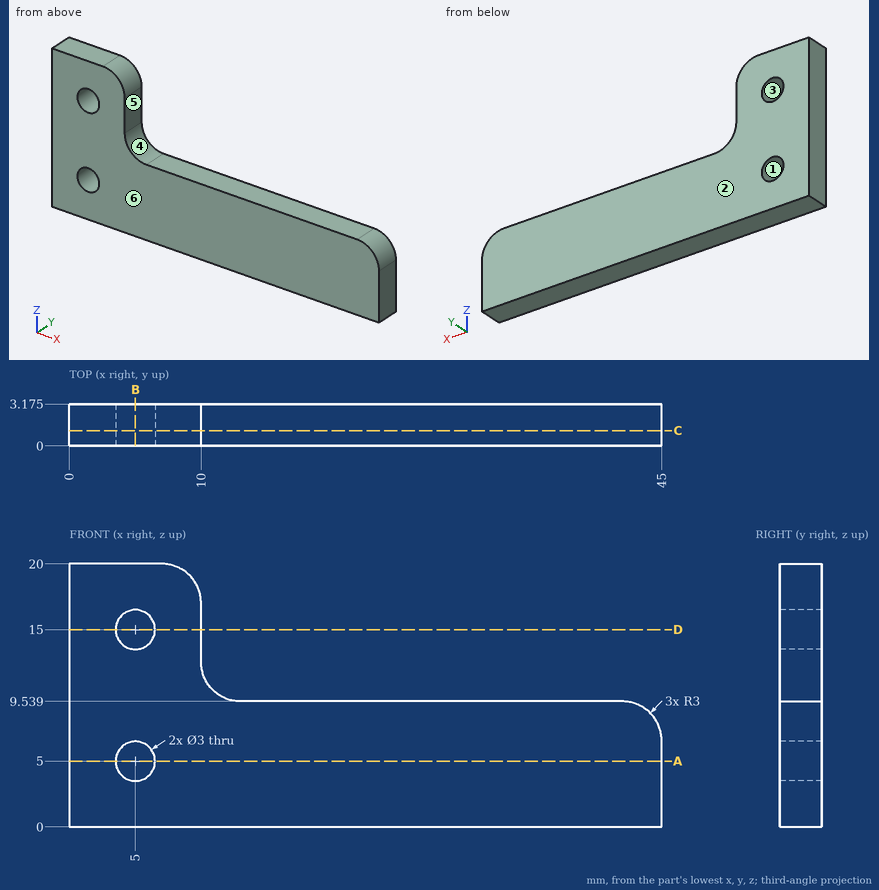
Study the drawing (mm; zero at the part's minimum x, y, z) and answer. A direction names the side the tool comes from. Give positions to 0.01 mm unless a question says otherwise; leave off trailing zeros. Write each loop counter-clockwise with the first axis right and the second up, starting at its lowest first coordinate (ties: lowest second). Pieces come first, ordered by that corner, then holes. Notation, with made-up numbers: (-39, 48.25) - (-15, 48.25) arc R13 ccw to (-15, 63.25) - close; hole circle Ø6 at (19.5, -8). An arc over 180 degrees is marked (long way). Use CSV: the item, a comma, the result in double quotes. Start each with the question number.
(1) Find section A-A (z = 5). Give the vertices of the cut face in (x, y) (1 decimal).
(2) Consider line 1 along Z through (x, y) = (5, 1.1); line 2 along Z through (x, y) = (4, 1.6); line 3 along Z through (x, y) = (41, 2). Determine where each line is inside the solid, lowest interval first.
(3) Find section B-B (x = 5). Give the vertices of the cut face in (y, z) (1 decimal).
(4) Find section D-D (z = 15). Give the vertices of the cut face in (x, y) (1 decimal), plus the area to 3 significant figures.
(5) Determine the mould class of the marked faces 1, 2, 3 and 4 for opening direction Z: +Z half, -Z half, draft (parallel to the pull), parting line (faces both ways), or undercut.
(6) Find section C-C (y = 1.15). Give the vertices of the cut face in (x, z).
(7) Given P1, Ø2.5, axis at x = 5, z = 5, coming from the +Y side; P2, Ø1, axis at x = 30.5, y = 1.5, coming from the +Z side; P3, Ø8, axis at x = 11.5, z = 10, coming from the -Y side; P4, Ø1.5, axis at y = 1, z = 11, coming from the +X side, each flat-ended and moving along its own axis, determine where each tip first touches the part or whether it passes through.
(8) For the marked faces 5 and 6, determine the directions among +Z, -Z, +X, -X, +Y, -Y from which every point of the face is accessible in a straight line to the end or side of a thin tool.
Findings below:
1,outline,"(0, 0) - (3.5, 0) - (3.5, 3.2) - (0, 3.2) - close; (6.5, 0) - (45, 0) - (45, 3.2) - (6.5, 3.2) - close"
2,line 1,"0 to 3.5, 6.5 to 13.5, 16.5 to 20"
2,line 2,"0 to 3.88, 6.12 to 13.88, 16.12 to 20"
2,line 3,"0 to 9.54"
3,outline,"(0, 0) - (3.2, 0) - (3.2, 3.5) - (0, 3.5) - close; (0, 6.5) - (3.2, 6.5) - (3.2, 13.5) - (0, 13.5) - close; (0, 16.5) - (3.2, 16.5) - (3.2, 20) - (0, 20) - close"
4,outline,"(0, 0) - (3.5, 0) - (3.5, 3.2) - (0, 3.2) - close; (6.5, 0) - (10, 0) - (10, 3.2) - (6.5, 3.2) - close"
4,area,"22.2 mm2"
5,face 1,"undercut"
5,face 2,"draft"
5,face 3,"undercut"
5,face 4,"+Z half"
6,outline,"(0, 0) - (45, 0) - (45, 6.54) arc R3 ccw to (42, 9.54) - (13, 9.54) arc R3 cw to (10, 12.54) - (10, 17) arc R3 ccw to (7, 20) - (0, 20) - close; hole circle Ø3 at (5, 5); hole circle Ø3 at (5, 15)"
7,P1,"through"
7,P2,"z = 9.54"
7,P3,"y = 0"
7,P4,"x = 11.06"
8,face 5,"+Z, +X, +Y, -Y"
8,face 6,"+Z, -Z, +X, -X, -Y"
